Study the drawing (mm; zero at the part's minimum x, y, z) and answer. A direction names the side the tool comes from. Coordinates: 2 decimals unless noted, no trailing zeros. Loops run counter-clockwise (first coordinate to the right, second up) from the corner with the lowest first, then second, coordinate; pieces in that order, holes last. Notation, with made-up numbers: (58, 45) - (107, 45) arc R26 cw to (107, 63) - close; hole circle Ø6 at (59.25, 23). An arc over 180 degrees is marked (long way). One line per item, written item: value. Start each with the question number.
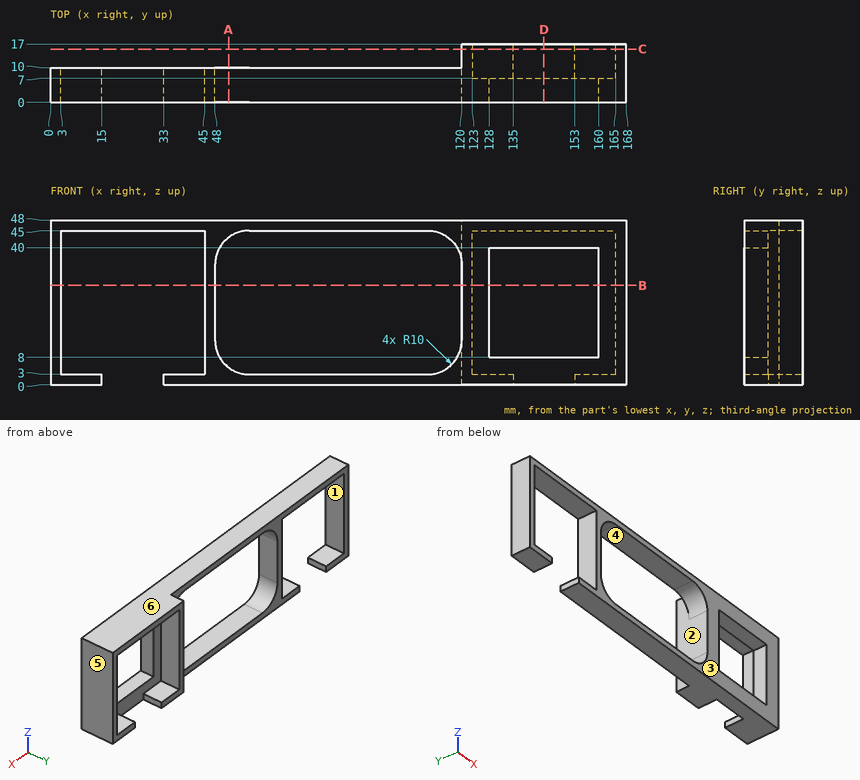
1) Section B-B, the plane z = 29 is taken. Determine the outline of the cut face in (x, y), and give its area (3 significant figures).
2) Section A-A, the plane x = 52 is taken. Determine the outline of the cut face in (y, z).
3) Section D-D, the plane x = 144 is taken. Determine the outline of the cut face in (y, z).
4) For the marked faces 1, 2 and 3, determine the directions among +Z, -Z, +X, -X, +Y, -Y from which every point of the face is accessible in a straight line to the end or side of a thin tool.
5) Straight lines are drawn through the part: L1, parallel to X at y = 6.25, z = 28; L2, parallel to X at y = 8.25, z = 17; L3, parallel to X at y = 13, z = 14.5. For each, find the intervals that lie inside material, in ascending order.
6) A flat-ended cylindrical pin translates along its axis: P1, Ø4, axis at y = 12.5, z = 11, coming from the -X side. Find the tip coordinate at first contact, or state that the pin passes through.
7) Determine the mould class of the marked faces 4, 5 and 6 for opening direction X: released by +X, released by -X, zero draft, split by the parting line, or undercut.
8) Section C-C, the plane y = 15.5 is taken. Determine the outline of the cut face in (x, z).
Answer below:
1. outline: (0, 0) - (3, 0) - (3, 10) - (0, 10) - close; (45, 0) - (48, 0) - (48, 10) - (45, 10) - close; (120, 0) - (128, 0) - (128, 7) - (123, 7) - (123, 17) - (120, 17) - close; (160, 0) - (168, 0) - (168, 17) - (165, 17) - (165, 7) - (160, 7) - close
1. area: 232 mm2
2. outline: (0, 0) - (10, 0) - (10, 5) - (0, 5) - close; (0, 43) - (10, 43) - (10, 48) - (0, 48) - close
3. outline: (0, 0) - (7, 0) - (7, 8) - (0, 8) - close; (0, 40) - (7, 40) - (7, 45) - (17, 45) - (17, 48) - (0, 48) - close
4. face 1: +Y, -Y
4. face 2: +Y
4. face 3: +Z, -Z, +X, -X, -Y
5. L1: 0 to 3, 45 to 48, 120 to 128, 160 to 168
5. L2: 0 to 3, 45 to 48, 120 to 123, 165 to 168
5. L3: 120 to 123, 165 to 168
6. P1: x = 120
7. face 4: undercut
7. face 5: released by +X
7. face 6: zero draft
8. outline: (120, 0) - (135, 0) - (135, 3) - (123, 3) - (123, 45) - (165, 45) - (165, 3) - (153, 3) - (153, 0) - (168, 0) - (168, 48) - (120, 48) - close
